Geometry check sheet. Reference: the model listing, model coordinates, mm. A direction names the side the tool comes from. Round coordinates to 2 decimals unless told otherwise and drop trailing zeros. Return JSON: item names as keys, results as strings. Group by question number.
from build123d import *

# Parameters (mm, degrees)
SKETCH1_R           = 3.175
BOSS_EXTRUDE1_DEPTH = 6.35
FILLET2_R           = 12.7
FILLET3_R           = 2.116666667


with BuildPart() as part:
    # Sketch1 → Boss-Extrude1 (new body)
    with BuildSketch(Plane(origin=(0, 0, 0), x_dir=(1, 0, 0), z_dir=(0, 1, 0))):
        with BuildLine():
            Line((12.7, 31.205256121), (-12.7, 31.205256121))
            Line((-12.7, 31.205256121), (-12.7, 4.715768363))
            Line((-12.7, 4.715768363), (-71.842048969, -54.426280605))
            Line((-71.842048969, -54.426280605), (-53.881536726, -72.386792847))
            Line((-53.881536726, -72.386792847), (8.980256121, -9.525))
            ThreePointArc((8.980256121, -9.525), (11.733270063, -5.40482347), (12.7, -0.544743879))
            Line((12.7, -0.544743879), (12.7, 31.205256121))
        make_face()
        with Locations(Location((-53.881536726, -54.426280605, 0), (0, 0, 270))):
            Circle(SKETCH1_R, mode=Mode.SUBTRACT)
        with Locations(Location((0, -0.544743879, 0), (0, 0, 270))):
            Circle(SKETCH1_R, mode=Mode.SUBTRACT)
        with Locations(Location((0, 18.505256121, 0), (0, 0, 270))):
            Circle(SKETCH1_R, mode=Mode.SUBTRACT)
    extrude(amount=BOSS_EXTRUDE1_DEPTH)

    # Fillet2
    fillet2_edges = [part.edges().sort_by_distance(p)[0] for p in [
        (12.7, 3.175, -31.205256121),
        (-12.7, 3.175, -31.205256121),
        (-71.842048969, 3.175, 54.426280605),
        (-53.881536726, 3.175, 72.386792847),
    ]]
    fillet(fillet2_edges, radius=FILLET2_R - 0.0001)  # a hair under: the kernel refuses the full size

    # Fillet3
    fillet3_edges = [part.edges().sort_by_distance(p)[0] for p in [
        (11.733270063, 6.35, 5.40482347),
        (-37.780931779, 0, 20.365163416),
        (-12.7, 0, -11.610562242),
        (12.7, 0, -8.980306121),
        (11.733270063, 0, 5.40482347),
        (12.7, 6.35, -8.980306121),
        (-12.7, 6.35, -11.610562242),
        (-37.780931779, 6.35, 20.365163416),
        (-17.960547597, 0, 36.465803719),
        (-53.881536726, 0, 67.126322027),
        (-66.581578148, 0, 54.426280605),
        (-8.98028541, 0, -27.485541531),
        (8.98028541, 0, -27.485541531),
        (-17.960547597, 6.35, 36.465803719),
        (-53.881536726, 6.35, 67.126322027),
        (-66.581578148, 6.35, 54.426280605),
        (-8.98028541, 6.35, -27.485541531),
        (8.98028541, 6.35, -27.485541531),
    ]]
    fillet(fillet3_edges, radius=FILLET3_R)


solid = part.part
1) Go/stop test with flat-tipped pins: P1, Ø4, axis at x = 0, z = 0.54, coming from the +Y side; P2, Ø1.5, axis at x = -26.5, y = 4.5, coming from the +Z side; P3, Ø2, axis at y = 4.5, z = 41.5, coming from the -X side; P4, Ø1, axis at y = 2.5, z = 7.5, coming from the +X side. Record where each tip stops, or that it passes through.
2) Sectioned sample at A-A on x = -1.5. State how many separate pieces and enclosed holes the cut face has, and give its area (3 significant figures).
3) Tool access check on faces 5 (the face through (12.06, 0.6, -9.11)), 6 (the face through (-12.7, 3, -12)). Record the directions out of +Z, -Z, +X, -X, +Y, -Y that give a thin tool (end or side, any length) a straight path to the whole face; none if there is none.
4) Material ranges on probe 1 along X at (y, z) = (5, -2); probe 2 along Z at (x, y) = (-51, 4.5); probe 3 along X at (y, z) = (5.5, 51.5), recorded low to high. Write a range as [from, to].
5) Mould release check, pull along X, two halves, no side actions. Record for faces 1 (the face through (-56.98, 3.13, 53.74)), 2 (the face through (-53.742, 3.19, 67.126)), 3 (the face through (8.881, 3.19, -27.584)), 4 (the face through (-66.58, 3.19, 54.29)): +X half, -X half, draft (parallel to the pull), parting line (faces both ways), or undercut.
Evaluation:
{
 "1": {"P1": "passes through", "P2": "stops at z = 45.74", "P3": "stops at x = -59.9", "P4": "stops at x = 10.94"},
 "2": {"separate pieces": "3", "enclosed holes": "0", "area": "249 mm2"},
 "3": {"face 5": "+Z, -Z, +X, -Y", "face 6": "-Z, -X, +Y, -Y"},
 "4": {"probe 1": "x = [-15.21, -1.9], [1.9, 12.56]", "probe 2": "z = [33.61, 53.09], [55.76, 66.78]", "probe 3": "x = [-65.81, -55.11], [-52.65, -33.59]"},
 "5": {"face 1": "undercut", "face 2": "parting line", "face 3": "+X half", "face 4": "-X half"}
}
